from build123d import *

# Parameters (mm, degrees)
F0_W     = 236.196054
F0_H     = 25
F1_DEPTH = 5
F2_R     = 2.5
F3_DEPTH = 20


with BuildPart() as f1:
    # F0 (on Front) → F1 (new body)
    with BuildSketch(Plane.XZ):
        with Locations((118.098027, 12.5)):
            Rectangle(F0_W, F0_H)
    extrude(amount=-F1_DEPTH)

    # F2 (on face) → F3 (join)
    with BuildSketch(Plane.XZ):
        with Locations((19.984195, 12.5)):
            Circle(F2_R)
        with Locations((50.584195, 12.5)):
            Circle(F2_R)
        with Locations((80.884195, 12.5)):
            Circle(F2_R)
        with Locations((117.244195, 12.5)):
            Circle(F2_R)
    extrude(amount=F3_DEPTH)


solid = f1.part
Input: part model. Units: mm. Frame: model coordinates. A direction names the side the tool comes from. Round coordinates to 2 decimals unless told otherwise and drop trailing zeros. Order: outer loops, then holes, each group sorted by start corner. A loop starts at its lowest first (then second) coordinate and runs counter-clockwise, first axis right, second up.
1. Cut plane C-C, the plane x = 186. Output: boundary loops of the cut face in (y, z), then the cut area to 3 significant figures.
The answers:
outline: (0, 0) - (5, 0) - (5, 25) - (0, 25) - close
area: 125 mm2
2. Mould query, pull axis X, two halves, no side actions, for faces 3 (the face through (48.6, -9.86, 10.98)), 4 (the face through (117, -20, 13)), 5 (the face through (0, 2, 12)). Classes: released by +X, released by -X, zero draft, split by the parting line, or undercut.
The answers:
face 3: undercut
face 4: zero draft
face 5: released by -X
3. Cut plane B-B, the plane z = 12.5. Output: boundary loops of the cut face in (x, y), then the cut area to 3 significant figures.
The answers:
outline: (0, 0) - (17.48, 0) - (17.48, -20) - (22.48, -20) - (22.48, 0) - (48.08, 0) - (48.08, -20) - (53.08, -20) - (53.08, 0) - (78.38, 0) - (78.38, -20) - (83.38, -20) - (83.38, 0) - (114.74, 0) - (114.74, -20) - (119.74, -20) - (119.74, 0) - (236.2, 0) - (236.2, 5) - (0, 5) - close
area: 1,580 mm2
4. Set-up query: faces 1 (the face through (81, -20, 13)), 2 (the face through (78.9, -9.86, 10.98)). Return all of +Z, -Z, +X, -X, +Y, -Y with unobstructed straight access to the full face (end or side cutting, diameter ignored); none if empty.
The answers:
face 1: +Z, -Z, +X, -X, -Y
face 2: -Y
5. Cut plane A-A, the plane y = -14.75. Output: boundary loops of the cut face in (x, z), then the cut area to 3 significant figures.
The answers:
outline: circle Ø5 at (19.98, 12.5); circle Ø5 at (50.58, 12.5); circle Ø5 at (80.88, 12.5); circle Ø5 at (117.24, 12.5)
area: 78.5 mm2
6. Pin query (flat end, axial travel): P1, Ø3, axis at y = -8, z = 14.5, coming from the +X side. Return the tip coordinate at first contact, or that it passes through.
The answers:
P1: stops at x = 119.69
7. Material intervals for line 1 (X direction, y = -17.25, z = 11.75); line 2 (X direction, y = -14.25, z = 10.5); line 3 (Y direction, x = 152, z = 20.75), sorted ascending.
The answers:
line 1: x = 17.6 to 22.37, 48.2 to 52.97, 78.5 to 83.27, 114.86 to 119.63
line 2: x = 18.48 to 21.48, 49.08 to 52.08, 79.38 to 82.38, 115.74 to 118.74
line 3: y = 0 to 5
